The listing builds one solid part. Answer for the finished solid, in the listing's coordinates (mm). Face numbers are marked on the shaded views. Coordinates: 2 decimals unless noted, no trailing zeros. Loops run counter-clockwise (first coordinate to the right, second up) from the corner with the lowest first, then second, coordinate; pieces in that order, holes last. Notation, with made-up numbers: (19, -35) - (77, -35) arc R18 ccw to (77, -16) - close; hole circle Ø7 at (84.25, 85.25). An arc over 180 degrees is marked (long way). Write each question's results on one line, items separated by ' | '. Start each with the question number.
(1) Find section A-A on x = 0. Determine the outline of the cut face in (y, z), then the cut area to 3 significant figures.
(2) Consider line 1 (X direction, y = 39, z = 0.5); line 2 (X direction, y = 30, z = 9.5); line 3 (Z direction, x = -5.5, y = 134). Determine where each line is inside the solid, lowest interval first. Write a range as from..to.
(3) Given pin 1 Ø2 at (y, z) = (87.5, -5.5) entering from -X; pin 2 Ø4 at (y, z) = (53, 10.5) entering from +X; pin 3 Ø12 at (x, y) = (-11, 70) entering from -Z, each flat-ended and moving along its own axis, determine where each tip first touches the part or whether it passes through.
(4) Determine the mould class of the marked faces 1 and 2 for opening direction Z: released by +Z, released by -Z, zero draft, split by the parting line, or undercut.
(5) Find section C-C on y = 37. Determine the outline of the cut face in (x, z).
(6) Find section B-B on z = 0. Determine the outline of the cut face in (x, y), then the cut area to 3 significant figures.
from build123d import *

# Parameters (mm, degrees)
SKETCH1_R           = 14.5
BASE_DEPTH          = 186.69
TOP_FILLET_R        = 4.365625
CASING_WALLS_T      = -1.5
SKETCH2_R           = 10.25
TOP_HOLE_DEPTH      = 188.812821995
TOP_HOLE_DEPTH_BACK = 188.812821995


with BuildPart() as part:
    # Sketch1 → base (new body)
    with BuildSketch(Plane(origin=(0, 0, 0), x_dir=(1, 0, 0), z_dir=(0, 1, 0))):
        with Locations(Location((0, 0, 0), (0, 0, 90))):
            Circle(SKETCH1_R)
    extrude(amount=BASE_DEPTH)

    # top-fillet
    top_fillet_edges = [part.edges().sort_by_distance(p)[0] for p in [
        (0, 186.69, 14.5),
    ]]
    fillet(top_fillet_edges, radius=TOP_FILLET_R)

    # casing-walls
    casing_walls_openings = [part.faces().sort_by_distance(p)[0] for p in [
        (0, 0, 0),
    ]]
    offset(amount=CASING_WALLS_T, openings=casing_walls_openings, kind=Kind.INTERSECTION)

    # Sketch2 → top-hole (cut, two sides)
    with BuildSketch(Plane(origin=(0, 0, 0), x_dir=(1, 0, 0), z_dir=(0, 1, 0))) as top_hole_sk:
        with Locations(Location((0, 0, 0), (0, 0, 270))):
            Circle(SKETCH2_R)
    extrude(amount=TOP_HOLE_DEPTH, mode=Mode.SUBTRACT)
    extrude(top_hole_sk.sketch, amount=-TOP_HOLE_DEPTH_BACK, mode=Mode.SUBTRACT)


solid = part.part
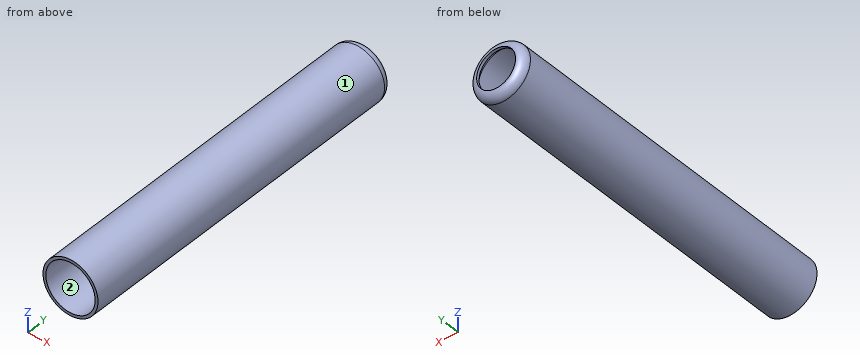
Values:
1) outline: (0, -14.5) - (182.32, -14.5) arc R4.37 ccw to (186.69, -10.25) - (185.19, -10.25) arc R2.87 cw to (182.32, -13) - (0, -13) - close; (0, 13) - (182.32, 13) arc R2.87 cw to (185.19, 10.25) - (186.69, 10.25) arc R4.37 ccw to (182.32, 14.5) - (0, 14.5) - close | area: 564 mm²
2) line 1: x = -14.49..-12.99, 12.99..14.49 | line 2: x = -10.95..-8.87, 8.87..10.95 | line 3: z = -13.42..-11.78, 11.78..13.42
3) pin 1: stops at x = -13.78 | pin 2: stops at x = 11.75 | pin 3: stops at z = -13.61
4) face 1: split by the parting line | face 2: undercut
5) outline: circle Ø29 at (0, 0); hole circle Ø26 at (0, 0)
6) outline: (-14.5, 0) - (-13, 0) - (-13, 182.32) arc R2.87 cw to (-10.25, 185.19) - (-10.25, 186.69) arc R4.37 ccw to (-14.5, 182.32) - close; (10.25, 185.19) arc R2.87 cw to (13, 182.32) - (13, 0) - (14.5, 0) - (14.5, 182.32) arc R4.37 ccw to (10.25, 186.69) - close | area: 564 mm²
